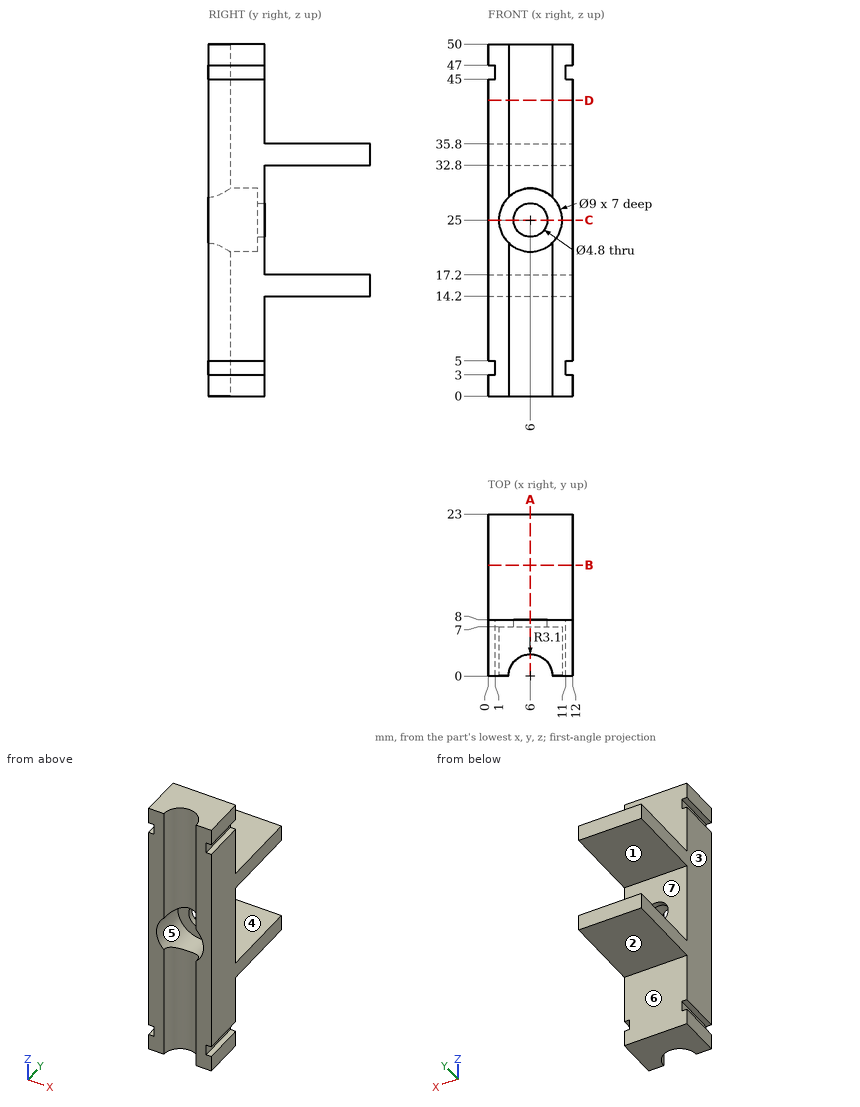
For this review, use the dimensioned drawing (mm, ordinates from the lowest corner) and the shaded views. A direction names the side the tool comes from. Coordinates: 2 decimals unless noted, no trailing zeros. Write each loop counter-clockwise with the first axis right and the second up, starting at its lowest first coordinate (ties: lowest second). Pieces come first, ordered by that corner, then holes. Notation, with made-up numbers: (44.25, 41.5) - (75.25, 41.5) arc R18 cw to (75.25, 69.5) - close; hole circle Ø2 at (24, 58.25). An arc over 180 degrees is marked (long way). Answer in a Markdown table with one row per item. Add a question column.
Q1. Consider section B-B on y = 15.75. Give the boundary of the cut face in (x, z).
Q2. Consider section A-A on x = 6. Give the boundary of the cut face in (y, z), then the cut area to 3 significant figures.
Q3. Consider section C-C on z = 25. Give the boundary of the cut face in (x, y), then the cut area to 3 significant figures.
Q4. Consider section D-D on z = 42. Give the boundary of the cut face in (x, y).
Q5. To check wall thickness, follow line 1 along Z through (x, y) = (3, 10); line 2 along Z through (x, y) = (6, 5.75); line 3 along Y through (x, z) = (3.5, 27). State the ranges of each line that lie inside material, in increasing order. Write a range as from..to.
Q6. Draft analysis for pull direction Z (two halves, no side actions). For the marked faces 1, 2, 3 and 4, state which applies: +Z half, -Z half, draft (parallel to the pull), parting line (faces both ways), or undercut.
Q7. For the marked faces 5, 6 and 7, list the 3-axis set-ups (+Z, -Z, +X, -X, +Y, -Y) from which the entire face can be reached by the end or side of a thin tool; tool diameter is ignored.
Q8. Clearance check with flat-ended pins moving along their axes: pin 1 (6 mm diameter, centred on x = 4.5, z = 7.5, fed in from +Y); pin 2 (1.5 mm diameter, centred on x = 5.5, y = 19.5, fed in from +Z); pin 3 (0.6 mm diameter, centred on y = 2.5, z = 4.5, fed in from +X). State where each tip first meets the part, or that it passes through.
Answers below:
| question | item | result |
|---|---|---|
| 1 | outline | (0, 14.2) - (12, 14.2) - (12, 17.2) - (0, 17.2) - close; (0, 32.8) - (12, 32.8) - (12, 35.8) - (0, 35.8) - close |
| 2 | outline | (3.1, 0) - (8, 0) - (8, 14.2) - (23, 14.2) - (23, 17.2) - (8, 17.2) - (8, 22.6) - (7, 22.6) - (7, 20.5) - (3.1, 20.5) - close; (3.1, 29.5) - (7, 29.5) - (7, 27.4) - (8, 27.4) - (8, 32.8) - (23, 32.8) - (23, 35.8) - (8, 35.8) - (8, 50) - (3.1, 50) - close |
| 2 | area | 295 mm² |
| 3 | outline | (0, 0) - (1.5, 0) - (1.5, 7) - (3.6, 7) - (3.6, 8) - (0, 8) - close; (8.4, 7) - (10.5, 7) - (10.5, 0) - (12, 0) - (12, 8) - (8.4, 8) - close |
| 3 | area | 28.2 mm² |
| 4 | outline | (0, 0) - (2.9, 0) arc R3.1 cw to (9.1, 0) - (12, 0) - (12, 8) - (0, 8) - close |
| 5 | line 1 | 14.2..17.2, 32.8..35.8 |
| 5 | line 2 | 0..20.5, 29.5..50 |
| 5 | line 3 | 7..8 |
| 6 | face 1 | undercut |
| 6 | face 2 | -Z half |
| 6 | face 3 | draft |
| 6 | face 4 | undercut |
| 7 | face 5 | -Y |
| 7 | face 6 | -Z, +X, -X, +Y |
| 7 | face 7 | +X, -X, +Y |
| 8 | pin 1 | y = 8 |
| 8 | pin 2 | z = 35.8 |
| 8 | pin 3 | x = 11 |
